```python
from build123d import *

# Parameters (mm, degrees)
SKETCH1_R             = 2.286
SKETCH1_R_2           = 7.366
BOSS_EXTRUDE1_DEPTH   = 15.494
CAVITY1_START         = 5.334
CAVITY1_OUTLINE_R     = 1.143
CAVITY1_OUTLINE_R_2   = 7.366
CAVITY1_OUTLINE_R_3   = 4.445
CAVITY1_DEPTH         = 10.16
CAVITY1_START_2       = 2.286
CAVITY1_2_OUTLINE_R   = 1.143
CAVITY1_2_OUTLINE_R_2 = 4.445
CAVITY1_2_DEPTH       = 3.048
CAVITY1_3_OUTLINE_R   = 1.905
CAVITY1_3_DEPTH       = 3.302
CAVITY1_START_3       = 13.716
CAVITY1_4_DEPTH       = 1.778
CAVITY1_START_4       = 4.064
CAVITY1_5_OUTLINE_R   = 2.286
CAVITY1_5_DEPTH       = 1.27
CAVITY1_START_5       = 2.032
CAVITY1_6_DEPTH       = 0.254
CHAMFER1_SIZE         = 1.27
CHAMFER1_SIZE2        = 29.087782247
FILLET1_R             = 10


# Read off the part's stored shape, not the designer's step: Cavity1
with BuildPart() as part:
    # Sketch1 → Boss-Extrude1 (new body)
    with BuildSketch(Plane.XY):
        Polygon((-10.16, 10.16), (-27.94, -34.29), (-43.18, -91.44), (-43.18, -116.84), (10.16, -116.84), (10.16, 10.16), align=None)
        Circle(SKETCH1_R, mode=Mode.SUBTRACT)
        with Locations((-6.35, -76.2)):
            Circle(SKETCH1_R_2, mode=Mode.SUBTRACT)
        with Locations((-7.228672556, -27.94)):
            Circle(SKETCH1_R, mode=Mode.SUBTRACT)
        with Locations((-19.928672556, -27.94)):
            Circle(SKETCH1_R, mode=Mode.SUBTRACT)
        with Locations((5.471327444, -27.94)):
            Circle(SKETCH1_R, mode=Mode.SUBTRACT)
    extrude(amount=BOSS_EXTRUDE1_DEPTH)

    # Cavity1 outline → Cavity1 (cut)
    # profile 1 of 6: a face of its own
    with BuildSketch(Plane.XY.offset(CAVITY1_START)):
        with Locations((7.62, -85.344)):
            Circle(CAVITY1_OUTLINE_R)
    # profile 2 of 6: a face of its own
    with BuildSketch(Plane.XY.offset(CAVITY1_START)):
        with BuildLine():
            ThreePointArc((3.714128852, -86.430567503), (8.001, -76.2), (3.714128852, -65.969432496))
            ThreePointArc((3.714128852, -65.969432496), (3.886847552, -62.160894786), (0.313505747, -63.489811482))
            ThreePointArc((0.313505747, -63.489811482), (-6.35, -61.849), (-13.013505747, -63.489811482))
            ThreePointArc((-13.013505747, -63.489811482), (-16.586847552, -62.160894786), (-16.414128852, -65.969432496))
            ThreePointArc((-16.414128852, -65.969432496), (-20.701, -76.2), (-16.414128852, -86.430567503))
            ThreePointArc((-16.414128852, -86.430567503), (-16.586847552, -90.239105214), (-13.013505747, -88.910188518))
            ThreePointArc((-13.013505747, -88.910188518), (-6.35, -90.551), (0.313505747, -88.910188518))
            ThreePointArc((0.313505747, -88.910188518), (3.886847552, -90.239105214), (3.714128852, -86.430567503))
        make_face()
        with Locations((-6.35, -76.2)):
            Circle(CAVITY1_OUTLINE_R_2, mode=Mode.SUBTRACT)
    # profile 3 of 6: a face of its own
    with BuildSketch(Plane.XY.offset(CAVITY1_START)):
        with Locations((7.62, -41.656)):
            Circle(CAVITY1_OUTLINE_R)
    # profile 4 of 6: a face of its own
    with BuildSketch(Plane.XY.offset(CAVITY1_START)):
        with Locations((-6.35, -50.8)):
            Circle(CAVITY1_OUTLINE_R_3)
    # profile 5 of 6: a face of its own
    with BuildSketch(Plane.XY.offset(CAVITY1_START)):
        with Locations((-20.32, -85.344)):
            Circle(CAVITY1_OUTLINE_R)
    # profile 6 of 6: a face of its own
    with BuildSketch(Plane.XY.offset(CAVITY1_START)):
        with Locations((-20.32, -41.656)):
            Circle(CAVITY1_OUTLINE_R)
    extrude(amount=CAVITY1_DEPTH, mode=Mode.SUBTRACT)

    # Cavity1 2 outline → Cavity1 2 (cut)
    with BuildSketch(Plane.XY.offset(CAVITY1_START_2)):
        with Locations((7.62, -85.344)):
            Circle(CAVITY1_2_OUTLINE_R)
        with Locations((7.62, -41.656)):
            Circle(CAVITY1_2_OUTLINE_R)
        with BuildLine():
            ThreePointArc((-9.97043784, -62.313185), (-6.35, -67.31), (-2.72956216, -62.313185))
            ThreePointArc((-2.72956216, -62.313185), (-6.35, -61.849), (-9.97043784, -62.313185))
        make_face()
        with Locations((-6.35, -50.8)):
            Circle(CAVITY1_2_OUTLINE_R_2)
        with Locations((-20.32, -85.344)):
            Circle(CAVITY1_2_OUTLINE_R)
        with Locations((-20.32, -41.656)):
            Circle(CAVITY1_2_OUTLINE_R)
    extrude(amount=CAVITY1_2_DEPTH, mode=Mode.SUBTRACT)

    # Cavity1 3 outline → Cavity1 3 (cut)
    with BuildSketch(Plane.XY):
        with Locations((7.62, -85.344)):
            Circle(CAVITY1_3_OUTLINE_R)
        with Locations((7.62, -41.656)):
            Circle(CAVITY1_3_OUTLINE_R)
        with Locations((-20.32, -85.344)):
            Circle(CAVITY1_3_OUTLINE_R)
        with Locations((-20.32, -41.656)):
            Circle(CAVITY1_3_OUTLINE_R)
    extrude(amount=CAVITY1_3_DEPTH, mode=Mode.SUBTRACT)

    # Cavity1 4 outline → Cavity1 4 (cut)
    with BuildSketch(Plane.XY.offset(CAVITY1_START_3)):
        with BuildLine():
            Line((-2.021487251, -51.810941334), (-0.080238237, -49.901274035))
            ThreePointArc((-0.080238237, -49.901274035), (-0.020091344, -49.399733991), (0, -48.895))
            ThreePointArc((0, -48.895), (-0.99932539, -45.475529103), (-3.682765738, -43.132330359))
            Line((-3.682765738, -43.132330359), (-4.827346661, -46.623931058))
            ThreePointArc((-4.827346661, -46.623931058), (-2.708144766, -48.2514876), (-1.905, -50.8))
            ThreePointArc((-1.905, -50.8), (-1.93421784, -51.308815207), (-2.021487251, -51.810941334))
        make_face()
        with BuildLine():
            ThreePointArc((-5.088099029, -55.118351664), (-1.768956382, -53.292333211), (-0.080238237, -49.901274035))
            Line((-0.080238237, -49.901274035), (-2.021487251, -51.810941334))
            ThreePointArc((-2.021487251, -51.810941334), (-3.122489186, -53.856337505), (-5.104913564, -55.067058093))
            Line((-5.104913564, -55.067058093), (-5.088099029, -55.118351664))
        make_face()
        with BuildLine():
            Line((-4.827346661, -46.623931058), (-3.682765738, -43.132330359))
            ThreePointArc((-3.682765738, -43.132330359), (-6.35, -42.545), (-9.017234262, -43.132330359))
            Line((-9.017234262, -43.132330359), (-7.872653339, -46.623931058))
            ThreePointArc((-7.872653339, -46.623931058), (-6.35, -46.355), (-4.827346661, -46.623931058))
        make_face()
        with BuildLine():
            ThreePointArc((-5.446692173, -55.180422418), (-5.266950842, -55.15195649), (-5.088099029, -55.118351664))
            Line((-5.088099029, -55.118351664), (-5.104913564, -55.067058093))
            ThreePointArc((-5.104913564, -55.067058093), (-5.256864048, -55.108489154), (-5.410186924, -55.144511064))
            Line((-5.410186924, -55.144511064), (-5.446692173, -55.180422418))
        make_face()
        with BuildLine():
            Line((-7.872653339, -46.623931058), (-9.017234262, -43.132330359))
            ThreePointArc((-9.017234262, -43.132330359), (-11.955544051, -45.911650223), (-12.619761763, -49.901274035))
            Line((-12.619761763, -49.901274035), (-10.678512749, -51.810941334))
            ThreePointArc((-10.678512749, -51.810941334), (-10.259642573, -48.6851194), (-7.872653339, -46.623931058))
        make_face()
        with BuildLine():
            ThreePointArc((-6.35, -55.245), (-5.897193393, -55.228835029), (-5.446692173, -55.180422418))
            Line((-5.446692173, -55.180422418), (-5.410186924, -55.144511064))
            ThreePointArc((-5.410186924, -55.144511064), (-5.877414917, -55.219806369), (-6.35, -55.245))
        make_face()
        with BuildLine():
            Line((-7.289813076, -55.144511064), (-7.253307826, -55.180422418))
            ThreePointArc((-7.253307826, -55.180422418), (-6.802806607, -55.228835029), (-6.35, -55.245))
            ThreePointArc((-6.35, -55.245), (-6.822585083, -55.219806369), (-7.289813076, -55.144511064))
        make_face()
        with BuildLine():
            ThreePointArc((-7.611900971, -55.118351664), (-7.433049158, -55.15195649), (-7.253307826, -55.180422418))
            Line((-7.253307826, -55.180422418), (-7.289813076, -55.144511064))
            ThreePointArc((-7.289813076, -55.144511064), (-7.443135952, -55.108489154), (-7.595086436, -55.067058093))
            Line((-7.595086436, -55.067058093), (-7.611900971, -55.118351664))
        make_face()
        with BuildLine():
            Line((-10.678512749, -51.810941334), (-12.619761763, -49.901274035))
            ThreePointArc((-12.619761763, -49.901274035), (-10.931043618, -53.292333211), (-7.611900971, -55.118351664))
            Line((-7.611900971, -55.118351664), (-7.595086436, -55.067058093))
            ThreePointArc((-7.595086436, -55.067058093), (-9.577510814, -53.856337505), (-10.678512749, -51.810941334))
        make_face()
    extrude(amount=CAVITY1_4_DEPTH, mode=Mode.SUBTRACT)

    # Cavity1 5 outline → Cavity1 5 (cut)
    with BuildSketch(Plane.XY.offset(CAVITY1_START_4)):
        with Locations((2.54, -88.392)):
            Circle(CAVITY1_5_OUTLINE_R)
        with Locations((2.54, -64.008)):
            Circle(CAVITY1_5_OUTLINE_R)
        with Locations((-15.24, -88.392)):
            Circle(CAVITY1_5_OUTLINE_R)
        with Locations((-15.24, -64.008)):
            Circle(CAVITY1_5_OUTLINE_R)
    extrude(amount=CAVITY1_5_DEPTH, mode=Mode.SUBTRACT)

    # Cavity1 6 outline → Cavity1 6 (cut)
    with BuildSketch(Plane.XY.offset(CAVITY1_START_5)):
        with BuildLine():
            ThreePointArc((-9.97043784, -62.313185), (-6.35, -67.31), (-2.72956216, -62.313185))
            ThreePointArc((-2.72956216, -62.313185), (-6.35, -61.849), (-9.97043784, -62.313185))
        make_face()
    extrude(amount=CAVITY1_6_DEPTH, mode=Mode.SUBTRACT)

    # Chamfer1
    chamfer1_edges = [part.edges().sort_by_distance(p)[0] for p in [
        (10.16, -116.84, 7.747),
    ]]
    chamfer1_side = [part.faces().sort_by_distance(p)[0] for p in [
        (-16.51, -116.84, 7.747),
    ]]
    chamfer(chamfer1_edges, length=CHAMFER1_SIZE, length2=CHAMFER1_SIZE2, reference=chamfer1_side[0])

    # Fillet1
    fillet1_edges = [part.edges().sort_by_distance(p)[0] for p in [
        (-10.16, 10.16, 7.747),
        (10.16, 10.16, 7.747),
        (8.89, -116.84, 7.747),
        (-43.18, -116.84, 7.747),
        (-43.18, -91.44, 7.747),
        (-27.94, -34.29, 7.747),
    ]]
    fillet(fillet1_edges, radius=FILLET1_R)


solid = part.part
```
Check sheet for the modelled part. Datum: model origin and axes. Units: mm. A direction names the side the tool comes from. Round coordinates to 2 decimals unless told otherwise and drop trailing zeros. Loops run counter-clockwise (first coordinate to the right, second up) from the corner with the lowest first, then second, coordinate; pieces in that order, holes last. Notation, with made-up numbers: (27.25, 51) -> (84.25, 51) arc R24 ccw to (84.25, 62) -> close; hole circle Ø6 at (37, 28.5). An arc over 180 degrees is marked (long way). Answer in a Markdown table with one row per item.
Q1. Sectioned sample at B-B on x = -26. Enter the section's corners in (y, z), then the cut area to 3 significant figures.
Data:
| item | result |
|---|---|
| outline | (-116.84, 0) -> (-29.44, 0) -> (-29.44, 15.49) -> (-116.84, 15.49) -> close |
| area | 1,350 mm^2 |
Q2. Release check for a two-part mould opening along Y. For faces 4 (the face through (7.31, 7.15, 7.86)), 5 (the face through (-11, -67, 0)), 6 (the face through (6.3, -114, 7.9)), 7 (the face through (0.454, -79.021, 2.63)) record: released by +Y, released by -Y, zero draft, split by the parting line, or undercut.
Data:
| item | result |
|---|---|
| face 4 | released by +Y |
| face 5 | zero draft |
| face 6 | released by -Y |
| face 7 | undercut |
Q3. Sectioned sample at A-A on y = -27.94. Enter the section's corners in (x, z).
Data:
| item | result |
|---|---|
| outline | (-25.4, 0) -> (-22.21, 0) -> (-22.21, 15.49) -> (-25.4, 15.49) -> close; (-17.64, 0) -> (-9.51, 0) -> (-9.51, 15.49) -> (-17.64, 15.49) -> close; (-4.94, 0) -> (3.19, 0) -> (3.19, 15.49) -> (-4.94, 15.49) -> close; (7.76, 0) -> (10.16, 0) -> (10.16, 15.49) -> (7.76, 15.49) -> close |
Q4. Sectioned sample at C-C on z = 10.5. Give the number of separate pieces and of enclosed holes in the cut face, then the cut area to 3 significant figures.
Data:
| item | result |
|---|---|
| separate pieces | 1 |
| enclosed holes | 10 |
| area | 4,340 mm^2 |
Q5. Thickness scan on L1, parallel to Y at x = -15.24, z = 4.3; L2, parallel to Y at x = -15.24, z = 8; L3, parallel to X at y = -29, z = 13.5. Record the ranges inside material, lowest first.
Data:
| item | result |
|---|---|
| L1 | y = -116.84 to -90.68, -86.11 to -66.29, -61.72 to -2.54 |
| L2 | y = -116.84 to -90.68, -61.72 to -2.54 |
| L3 | x = -25.82 to -21.95, -17.9 to -9.25, -5.2 to 3.45, 7.5 to 10.16 |
Q6. Set-up check for faces 1 (the face through (-20, -87, 3.302)), 2 (the face through (-20.7, -76, 10.3)), 3 (the face through (10.16, -44, 8)): record each of +Z, -Z, +X, -X, +Y, -Y from which the full face is reachable in a straight line by a thin tool's end or side.
Data:
| item | result |
|---|---|
| face 1 | -Z |
| face 2 | +Z |
| face 3 | +Z, -Z, +X, +Y, -Y |
Q7. Go/stop test with flat-tipped pins: P1, Ø1.9, axis at x = -20.5, y = -84.5, coming from the -Z side; P2, Ø8, axis at y = -61.5, z = 13.5, coming from the -X side; P3, Ø5, axis at x = -24, z = 4, coming from the +Y side. Record where each tip stops, or that it passes through.
Data:
| item | result |
|---|---|
| P1 | stops at z = 3.3 |
| P2 | stops at x = -36.26 |
| P3 | stops at y = -18.19 |
Q8. Sectioned sample at D-D on y = -76.2. Enter the section's corners in (x, z), then the cut area to 3 significant figures.
Data:
| item | result |
|---|---|
| outline | (-39.12, 0) -> (-13.72, 0) -> (-13.72, 5.33) -> (-20.7, 5.33) -> (-20.7, 15.49) -> (-39.12, 15.49) -> close; (1.02, 0) -> (10.16, 0) -> (10.16, 15.49) -> (8, 15.49) -> (8, 5.33) -> (1.02, 5.33) -> close |
| area | 393 mm^2 |
